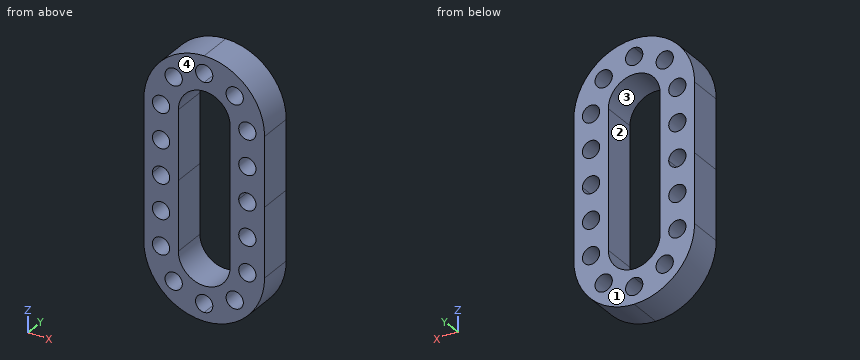
from build123d import *
from build123d import SkipClean  # not in build123d's __all__

# Parameters (mm, degrees)
F0_R     = 5
F1_DEPTH = 20


with BuildPart() as f1:
    # F0 (on Front) → F1 (new body)
    with BuildSketch(Plane.XZ):
        with BuildLine():
            Line((-15, 0), (-15, 40))
            ThreePointArc((-15, 40), (-10.6066017178, 50.6066017178), (0, 55))
            Line((0, 55), (0, 60))
            ThreePointArc((0, 60), (-5, 65), (0, 70))
            Line((0, 70), (0, 75))
            ThreePointArc((0, 75), (-24.7487373415, 64.7487373415), (-35, 40))
            Line((-35, 40), (-35, 0))
            Line((-35, 0), (-30, 0))
            ThreePointArc((-30, 0), (-25, 5), (-20, 0))
            Line((-20, 0), (-15, 0))
        make_face()
        with Locations((-25, 20)):
            Circle(F0_R, mode=Mode.SUBTRACT)
        with Locations((-25, 40)):
            Circle(F0_R, mode=Mode.SUBTRACT)
        with Locations((-17.6776695297, 57.6776695297)):
            Circle(F0_R, mode=Mode.SUBTRACT)
    extrude(amount=F1_DEPTH)

    # F2: F1 across plane


with BuildPart() as f1_1:
    add(f1.part, clean=False)
    with SkipClean():  # cleaning this boolean's faces spoils the solid; the shape is the same uncleaned
        add(f1.part.mirror(Plane.YZ), clean=False)

    # F3: F1 across plane


with BuildPart() as f1_2:
    add(f1_1.part, clean=False)
    with SkipClean():  # cleaning this boolean's faces spoils the solid; the shape is the same uncleaned
        add(f1_1.part.mirror(Plane.XY), clean=False)


solid = f1_2.part
Build history of the part. All positions in model axes, mm. Face numbers are marked on the shaded views. A direction names the side the tool comes from. Round coordinates to 2 decimals unless told otherwise and drop trailing zeros. Write each loop counter-clockwise with the first axis right and the second up, starting at its lowest first coordinate (ties: lowest second). Pieces come first, ordered by that corner, then holes. Notation, with made-up numbers: M 74.5,42.5 L 99.5,42.5 A19 cw 99.5,63.5 Z; hole C 25.25,-38.5 d5. An arc over 180 degrees is marked long. Use CSV: the item, a comma, the result in double quotes.
1. Saw through at B-B (x = -25). Give the cut face in (y, z).
Reply:
outline,"M -20,-64.49 L 0,-64.49 L 0,-45 L -20,-45 Z; M -20,-35 L 0,-35 L 0,-25 L -20,-25 Z; M -20,-15 L 0,-15 L 0,-5 L -20,-5 Z; M -20,5 L 0,5 L 0,15 L -20,15 Z; M -20,25 L 0,25 L 0,35 L -20,35 Z; M -20,45 L 0,45 L 0,64.49 L -20,64.49 Z"
2. Flat gauge pins, fed straight in: pin 1 (16 mm diameter, centred on x = -17.68, z = -57.68, fed in from +Y); pin 2 (8 mm diameter, centred on x = 25, z = 20, fed in from -Y); pin 3 (1 mm diameter, centred on x = 26, y = -5, fed in from -Z); pin 4 (5 mm diameter, centred on x = 12.5, y = -8, fed in from +Z). Where does each tip first touch, or does it go through?
Reply:
pin 1,"stops at y = 0"
pin 2,"passes through"
pin 3,"stops at z = -63.97"
pin 4,"stops at z = 73.54"
3. Two-plate mould, pull along X, no slides. Class the marked faces 1 and 2: +X half, -X half, draft (parallel to the pull), parting line (faces both ways), or undercut.
Reply:
face 1,"draft"
face 2,"undercut"
4. Tool access for the marked faces 3 and 4: list every direction of +Z, -Z, +X, -X, +Y, -Y with a clear straight run to the whole face (end or side of a thin tool).
Reply:
face 3,"+Y, -Y"
face 4,"+Z, -Z, +X, -X, -Y"
5. Saw through at A-A (z = -31.5). Give the cut face in (x, y).
Reply:
outline,"M -35,-20 L -15,-20 L -15,0 L -35,0 Z; M 15,-20 L 35,-20 L 35,0 L 15,0 Z"
6. Saw through at D-D (y = -15). State how many separate pieces and enclosed holes the cut face has, plus the area to 3 significant figures.
Reply:
separate pieces,"1"
enclosed holes,"17"
area,"5,080 mm²"
7. Wall check: probe 1 along X at (y, z) = (-5.5, -40); probe 2 along Z at (x, y) = (-18, -5); probe 3 along X at (y, z) = (-3.25, 58). Give the ranges that are in metal, low to high. Write a range as from..to.
Reply:
probe 1,"x = -35..-30, -20..-15, 15..20, 30..35"
probe 2,"z = -70.02..-62.67, -52.69..52.69, 62.67..70.02"
probe 3,"x = -30.02..-22.67, -12.69..12.69, 22.67..30.02"
8. Saw through at C-C (x = 18). Give the cut face in (y, z), plus the area to 3 significant figures.
Reply:
outline,"M -20,-70.02 L 0,-70.02 L 0,-62.67 L -20,-62.67 Z; M -20,-52.69 L 0,-52.69 L 0,52.69 L -20,52.69 Z; M -20,62.67 L 0,62.67 L 0,70.02 L -20,70.02 Z"
area,"2,400 mm²"
